The drawing under review shows one solid part. Ordinate dimensions are in mm from its lowest x, y, z. Round coordinates to 2 decimals unless told otherwise and drop trailing zeros. Write each loop counter-clockwise with the first axis right and the second up, starting at its lowest first coordinate (ties: lowest second). Pieces come first, ordered by that corner, then holes. Notation, with made-up numbers: (62, 34) -> (77, 34) arc R18 ccw to (77, 45) -> close; hole circle Ø5 at (60.25, -15.75). An arc over 180 degrees is marked (long way). Answer in a Markdown table with one row per item. Add a question column.
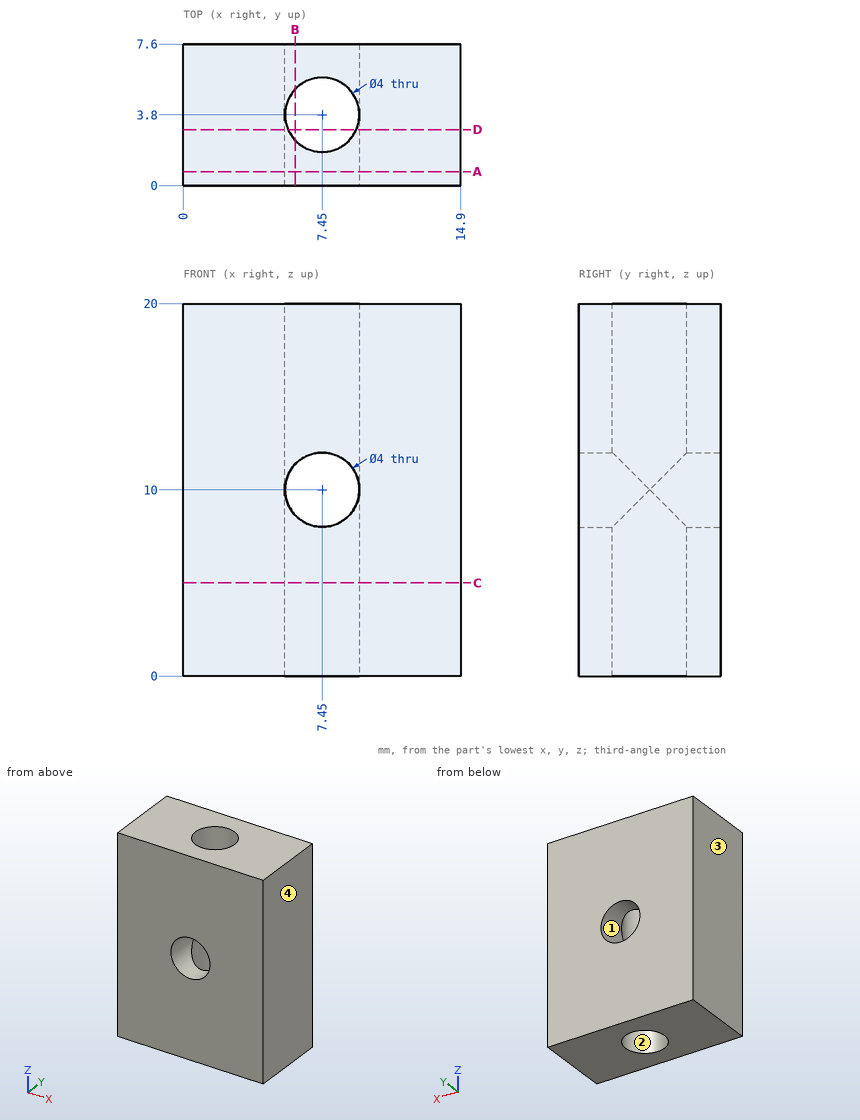
1. Add section B-B on x = 6. Write out the cut boundary in (y, z).
2. For L1, parallel to Z at x = 7.45, y = 5.85; L2, parallel to X at y = 3.8, z = 12.5; L3, parallel to Y at x = 7.45, z = 17.75, list the stretches that pass through material, from the lowest coordinate up.
3. Add section A-A on y = 0.75. Write out the cut boundary in (x, z), plus the area to 3 significant figures.
4. Add section D-D on y = 3. Write out the cut boundary in (x, z), plus the area to 3 significant figures.
5. Add section C-C on z = 5. Write out the cut boundary in (x, y).
6. Mouldability with a two-part tool opening along X and no side actions: class the marked faces 1, 2, 3 and 4 as pulls with the +X half, pulls with the -X half, needs draft (parallel to the pull), parting line crosses it, or undercut.
7. Insertion check: pin 1 Ø4 at (x, z) = (4, 3) entering from -Y. The pin has a flat end and moves straight along its axis. Give the tip position at first contact, or say it passes through.
Filled in:
| question | item | result |
|---|---|---|
| 1 | outline | (0, 0) -> (2.42, 0) -> (2.42, 8.62) -> (0, 8.62) -> close; (0, 11.38) -> (2.42, 11.38) -> (2.42, 20) -> (0, 20) -> close; (5.18, 0) -> (7.6, 0) -> (7.6, 8.62) -> (5.18, 8.62) -> close; (5.18, 11.38) -> (7.6, 11.38) -> (7.6, 20) -> (5.18, 20) -> close |
| 2 | L1 | 0 to 8, 12 to 20 |
| 2 | L2 | 0 to 5.45, 9.45 to 14.9 |
| 2 | L3 | 0 to 1.8, 5.8 to 7.6 |
| 3 | outline | (0, 0) -> (14.9, 0) -> (14.9, 20) -> (0, 20) -> close; hole circle Ø4 at (7.45, 10) |
| 3 | area | 285 mm² |
| 4 | outline | (0, 0) -> (5.62, 0) -> (5.62, 9.2) arc R2 cw to (5.62, 10.8) -> (5.62, 20) -> (0, 20) -> close; (9.28, 0) -> (14.9, 0) -> (14.9, 20) -> (9.28, 20) -> (9.28, 10.8) arc R2 cw to (9.28, 9.2) -> close |
| 4 | area | 224 mm² |
| 5 | outline | (0, 0) -> (14.9, 0) -> (14.9, 7.6) -> (0, 7.6) -> close; hole circle Ø4 at (7.45, 3.8) |
| 6 | face 1 | undercut |
| 6 | face 2 | undercut |
| 6 | face 3 | pulls with the -X half |
| 6 | face 4 | pulls with the +X half |
| 7 | pin 1 | y = 0 |
